```python
from build123d import *

# Parameters (mm, degrees)
SKETCH2_W         = 66.675
SKETCH2_H         = 85.3186
EXTRUDE1_DEPTH    = 24.6126
SKETCH3_OUTSIDE_W = 90.883
SKETCH3_OUTSIDE_H = 109.527
EXTRUDE2_DEPTH    = 24.6126
SKETCH4_OUTSIDE_W = 48.821
SKETCH4_OUTSIDE_H = 109.527
EXTRUDE3_DEPTH    = 67.675
FILLET1_R         = 1.5875
FILLET2_R         = 0.254
SKETCH5_R         = 4.0005
SKETCH5_R_2       = 1.1938
EXTRUDE4_DEPTH    = 67.675


with BuildPart() as part:
    # Sketch2 → Extrude1 (new body)
    with BuildSketch(Plane(origin=(0, 0, 0), x_dir=(0, 0, -1), z_dir=(1, 0, 0))):
        with Locations((33.3375, 42.6593)):
            Rectangle(SKETCH2_W, SKETCH2_H)
    extrude(amount=EXTRUDE1_DEPTH)

    # Sketch3 outside → Extrude2 (cut)
    with BuildSketch(Plane(origin=(24.6126, 0, 0), x_dir=(0, 0, -1), z_dir=(1, 0, 0))):
        with Locations((33.3375, 42.6595)):
            Rectangle(SKETCH3_OUTSIDE_W, SKETCH3_OUTSIDE_H)
        Polygon((1.5748, 85.3186), (1.5748, 9.1186), (9.1186, 1.5748), (57.5564, 1.5748), (65.1002, 9.1186), (65.1002, 85.3186), (66.675, 85.3186), (66.675, 8.466296482), (58.208703518, 0), (8.466296482, 0), (0, 8.466296482), (0, 85.3186), align=None, mode=Mode.SUBTRACT)
    extrude(amount=-EXTRUDE2_DEPTH, mode=Mode.SUBTRACT)

    # Sketch4 outside → Extrude3 (cut, through all)
    with BuildSketch(Plane.XY):
        with Locations((12.3065, 42.6595)):
            Rectangle(SKETCH4_OUTSIDE_W, SKETCH4_OUTSIDE_H)
        with BuildLine():
            Line((0, 73.0123), (0, 0))
            Line((0, 0), (24.6126, 0))
            Line((24.6126, 0), (24.6126, 73.0123))
            ThreePointArc((24.6126, 73.0123), (12.3063, 85.3186), (0, 73.0123))
        make_face(mode=Mode.SUBTRACT)
    extrude(amount=-EXTRUDE3_DEPTH, mode=Mode.SUBTRACT)

    # Fillet1
    fillet1_edges = [part.edges().sort_by_distance(p)[0] for p in [
        (12.3063, 8.466296482, -66.675),
        (12.3063, 0, -58.208703518),
        (12.3063, 0, -8.466296482),
        (12.3063, 8.466296482, 0),
    ]]
    fillet(fillet1_edges, radius=FILLET1_R)

    # Fillet2
    fillet2_edges = [part.edges().sort_by_distance(p)[0] for p in [
        (12.3063, 9.1186, -1.5748),
        (12.3063, 1.5748, -9.1186),
        (12.3063, 1.5748, -57.5564),
        (12.3063, 9.1186, -65.1002),
    ]]
    fillet(fillet2_edges, radius=FILLET2_R)

    # Sketch5 → Extrude4 (cut, through all)
    with BuildSketch(Plane.XY):
        with Locations((12.3063, 73.025)):
            Circle(SKETCH5_R)
        with Locations((12.3063, 81.3562)):
            Circle(SKETCH5_R_2)
        with Locations((3.9751, 73.025)):
            Circle(SKETCH5_R_2)
        with Locations((12.3063, 64.6938)):
            Circle(SKETCH5_R_2)
        with Locations((20.6375, 73.025)):
            Circle(SKETCH5_R_2)
    extrude(amount=-EXTRUDE4_DEPTH, mode=Mode.SUBTRACT)


solid = part.part
```
Check sheet for the modelled part. Datum: model origin and axes. Units: mm. A direction names the side the tool comes from. Give positions to 0.01 mm unless a question says otherwise; leave off trailing zeros. Write each loop counter-clockwise with the first axis right and the second up, starting at its lowest first coordinate (ties: lowest second). Pieces come first, ordered by that corner, then holes. Notation, with made-up numbers: (-30.5, 57.5) - (-10.5, 57.5) arc R23 cw to (-10.5, 71.5) - close; hole circle Ø7 at (4.25, 19). An arc over 180 degrees is marked (long way). Answer as a JSON object with one key per item and string values. Group by question number.
1) Thickness scan on probe 1 along Z at (x, y) = (21.25, 48.5) (3 decimals); probe 2 along Y at (x, z) = (15.75, -26); probe 3 along Y at (x, z) = (12.25, -4). Record the ranges inside material, lowest first. Write a range as from..to.
2) Sectioned sample at C-C (z = -20.5). Record the cut outline in (x, y).
3) Sectioned sample at B-B (x = 4.25). Give the number of separate pieces and of enclosed holes in the cut face, then the cut area to 3 significant figures.
4) Sectioned sample at A-A (y = 47.5). Record the cut outline in (x, z) (3 decimals).
5) Access from +Z, -Z, +X, -X, +Y, -Y to the whole of each face (thin tool, end or side, straight path). Record for faces 4 (the face through (12, 48, -1.575)), 5 (the face through (16.12, 74.23, -65.88)).
6) Release check for a two-part mould opening along Z. For faces 1 (the face through (12.479, 5.295, -61.277)), 2 (the face through (12.577, 85.316, -0.776)), 3 (the face through (12.479, 4.286, -62.495)) record: pulls with the +Z half, pulls with the -Z half, needs draft (parallel to the pull), parting line crosses it, or undercut.
7) Depth check by flat-ended pin: P1, Ø4, axis at x = 12.31, y = 81.36, coming from the -Z side (3 decimals); P2, Ø12.5, axis at x = 10.5, z = -28, coming from the +Y side; P3, Ø10, axis at x = 8, z = -56, coming from the +Y side. Enter the tip coordinate at first touch or a pass-through.
Geometry results:
{
 "1": {"probe 1": "z = -66.675..-65.1, -1.575..0", "probe 2": "y = 0..1.57", "probe 3": "y = 4.47..6.69"},
 "2": {"outline": "(0, 0) - (24.61, 0) - (24.61, 1.57) - (0, 1.57) - close"},
 "3": {"separate pieces": "3", "enclosed holes": "0", "area": "337 mm^2"},
 "4": {"outline": "(0, -66.675) - (24.613, -66.675) - (24.613, -65.1) - (0, -65.1) - close; (0, -1.575) - (24.613, -1.575) - (24.613, 0) - (0, 0) - close"},
 "5": {"face 4": "+X, -X, +Y", "face 5": "+Z, -Z"},
 "6": {"face 1": "undercut", "face 2": "needs draft", "face 3": "pulls with the -Z half"},
 "7": {"P1": "stops at z = -66.675", "P2": "stops at y = 1.57", "P3": "stops at y = 5.02"}
}
